Autodesk Inventor part; units mm, degrees
ref_plane "to_base_XY" through (0, -0.0254, 0) normal (0, 1, 0) x (1, 0, 0)
ref_plane "to_base_YZ" through (0, -0.0254, 0) normal (1, 0, 0) x (0, 0, -1)
ref_plane "to_base_ZX" through (0, -0.0254, 0) normal (0, 0, -1) x (0, 1, 0)
sketch "Sketch_2" plane through (0, 0, 0) normal (0, 1, 0) x (-1, 0, 0)
  line L0 (4.7037, -5.0719) -> (4.7037, 5.0719)
  arc A0 (4.7037, 5.0719) -> (4.5737, 5.2019) centre (4.5737, 5.0719) ccw
  line L1 (4.5737, 5.2019) -> (-4.5737, 5.2019)
  arc A1 (-4.5737, 5.2019) -> (-4.7037, 5.0719) centre (-4.5737, 5.0719) ccw
  line L2 (-4.7037, 5.0719) -> (-4.7037, -5.0719)
  arc A2 (-4.7037, -5.0719) -> (-4.5737, -5.2019) centre (-4.5737, -5.0719) ccw
  line L3 (-4.5737, -5.2019) -> (4.5737, -5.2019)
  arc A3 (4.5737, -5.2019) -> (4.7037, -5.0719) centre (4.5737, -5.0719) ccw
extrude "Extrusion1" add sketch "Sketch_2" along normal blind 0.254
sketch "Sketch_1" plane through (0, 0, -4.699) normal (0, 0, 1) x (1, 0, 0)
  line L0 (1.016, 0) -> (1.016, -1.016)
  line L1 (1.016, -1.016) -> (1.27, -1.016)
  line L2 (1.27, -1.016) -> (1.27, -2.4384)
  arc A0 (1.27, -2.4384) -> (2.413, -3.5814) centre (2.413, -2.4384) ccw
  line L3 (2.413, -3.5814) -> (10.0076, -3.5814)
  arc A1 (10.0076, -3.5814) -> (10.0076, -2.3114) centre (10.0076, -2.9464) ccw
  line L4 (10.0076, -2.3114) -> (3.048, -2.3114)
  arc A2 (2.54, -1.8034) -> (3.048, -2.3114) centre (3.048, -1.8034) ccw
  line L5 (2.54, -1.8034) -> (2.54, -1.016)
  line L6 (2.54, -1.016) -> (2.794, -1.016)
  line L7 (2.794, -1.016) -> (2.794, 0)
  line L8 (2.794, 0) -> (1.016, 0)
extrude "Extrusion2" add sketch "Sketch_1" along normal mid plane 0.762
pattern_linear "Rectangular Pattern1" count 3 spacing 4.699 along (0, 0, 1) of "Extrusion2"
sketch "Sketch_18" plane through (0, 0, -4.699) normal (0, 0, 1) x (1, 0, 0)
  line L0 (-2.794, 0) -> (-2.794, -1.016)
  line L1 (-2.794, -1.016) -> (-2.54, -1.016)
  line L2 (-2.54, -1.016) -> (-2.54, -6.3754)
  arc A0 (-2.54, -6.3754) -> (-1.524, -7.3914) centre (-1.524, -6.3754) ccw
  line L3 (-1.524, -7.3914) -> (10.0076, -7.3914)
  arc A1 (10.0076, -7.3914) -> (10.0076, -6.1214) centre (10.0076, -6.7564) ccw
  line L4 (10.0076, -6.1214) -> (-0.762, -6.1214)
  arc A2 (-1.27, -5.6134) -> (-0.762, -6.1214) centre (-0.762, -5.6134) ccw
  line L5 (-1.27, -5.6134) -> (-1.27, -1.016)
  line L6 (-1.27, -1.016) -> (-1.016, -1.016)
  line L7 (-1.016, -1.016) -> (-1.016, 0)
  line L8 (-1.016, 0) -> (-2.794, 0)
extrude "Extrusion3" add sketch "Sketch_18" along normal mid plane 0.762
pattern_linear "Rectangular Pattern2" count 3 spacing 4.699 along (0, 0, 1) of "Extrusion3"
ref_plane "to_base_XY" through (0, -0.0254, 0) normal (0, 1, 0) x (1, 0, 0)
ref_plane "to_base_YZ" through (0, -0.0254, 0) normal (1, 0, 0) x (0, 0, -1)
ref_plane "to_base_ZX" through (0, -0.0254, 0) normal (0, 0, -1) x (0, 1, 0)
properties part number "M202830_terminal_angW"
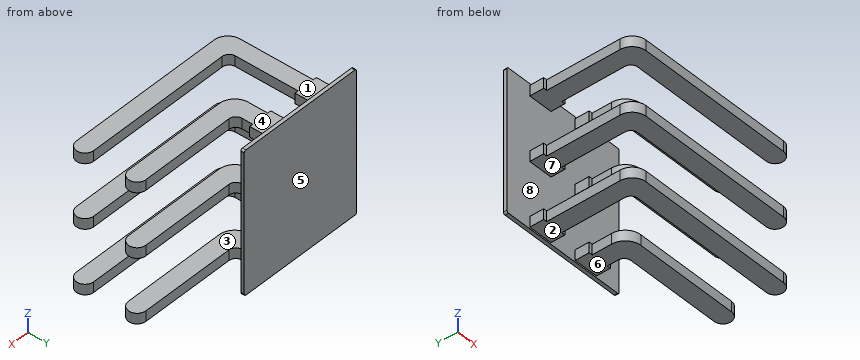
Build history of the part. All positions in model axes, mm. Face numbers are marked on the shaded views. A direction names the side the tool comes from. Coordinates: 2 decimals unless noted, no trailing zeros. Write each loop counter-clockwise with the first axis right and the second up, starting at its lowest first coordinate (ties: lowest second). Pieces come first, ordered by that corner, then holes. Notation, with made-up numbers: (-33.75, -1.75) -> (-20.75, -1.75) arc R18 ccw to (-20.75, 9.25) -> close; hole circle Ø7 at (-20.5, -4). An arc over 180 degrees is marked (long way). Use CSV: the item, a comma, the result in double quotes. Start each with the question number.
Q1. 3-axis set-ups, long thin cutter, end or side, ignore diameter. For the marked faces 4, 5, 6, 7 and 8: which of +Z, -Z, +X, -X, +Y, -Y reach the whole face in a straight line?
Q2. Cut at D-D, the plane z = 4.5. List the corners of the cut face in (x, y) (3 decimals).
Q3. Cut at A-A, the plane y = -5. List the corners of the cut face in (x, z).
Q4. Flat gauge pins, fed straight in: pin 1 Ø0.8 at (y, z) = (-3.5, 4.5) entering from +X; pin 2 Ø4 at (x, y) = (4, -2.5) entering from -Z; pin 3 Ø1 at (y, z) = (-1, -0.5) entering from -X. Where does each tip first touch, or does it go through?
Q5. Cut at C-C, the plane y = -1.5. List the corners of the cut face in (x, z).
Q6. Cut at B-B, the plane x = 9.5. List the corners of the cut face in (y, z), then the cut area to 3 significant figures.
Q7. Pull direction Z, two halves, no side cores. Call the marked faces 1, 2 and 3: released by +Z, released by -Z, zero draft, split by the parting line, or undercut.
Q8. Drill centre lines: probe 1 along Z at (x, y) = (9, -2.5); probe 2 along Y at (x, z) = (6.5, -0.25); probe 3 along Y at (x, z) = (-0.75, 4.5). Where is each one in solid material? Low to high.
Checked values:
1,face 4,"+Z, +X, -X, -Y"
1,face 5,"+Z, -Z, +X, -X, +Y"
1,face 6,"-Z, +X, -X, -Y"
1,face 7,"+X, -X, -Y"
1,face 8,"none"
2,outline,"(-4.704, 0) -> (-2.794, 0) -> (-2.794, -1.016) -> (-2.54, -1.016) -> (-2.54, -6.375) arc R1.016 ccw to (-1.524, -7.391) -> (10.008, -7.391) arc R0.635 ccw to (10.008, -6.121) -> (-0.762, -6.121) arc R0.508 cw to (-1.27, -5.613) -> (-1.27, -1.016) -> (-1.016, -1.016) -> (-1.016, 0) -> (1.016, 0) -> (1.016, -1.016) -> (1.27, -1.016) -> (1.27, -2.438) arc R1.143 ccw to (2.413, -3.581) -> (10.008, -3.581) arc R0.635 ccw to (10.008, -2.311) -> (3.048, -2.311) arc R0.508 cw to (2.54, -1.803) -> (2.54, -1.016) -> (2.794, -1.016) -> (2.794, 0) -> (4.704, 0) -> (4.704, 0.254) -> (-4.704, 0.254) -> close"
3,outline,"(-2.54, -5.08) -> (-1.27, -5.08) -> (-1.27, -4.32) -> (-2.54, -4.32) -> close; (-2.54, -0.38) -> (-1.27, -0.38) -> (-1.27, 0.38) -> (-2.54, 0.38) -> close; (-2.54, 4.32) -> (-1.27, 4.32) -> (-1.27, 5.08) -> (-2.54, 5.08) -> close"
4,pin 1,"stops at x = 10.62"
4,pin 2,"stops at z = -5.08"
4,pin 3,"stops at x = -2.79"
5,outline,"(-2.54, -5.08) -> (-1.27, -5.08) -> (-1.27, -4.32) -> (-2.54, -4.32) -> close; (-2.54, -0.38) -> (-1.27, -0.38) -> (-1.27, 0.38) -> (-2.54, 0.38) -> close; (-2.54, 4.32) -> (-1.27, 4.32) -> (-1.27, 5.08) -> (-2.54, 5.08) -> close; (1.27, -5.08) -> (2.54, -5.08) -> (2.54, -4.32) -> (1.27, -4.32) -> close; (1.27, -0.38) -> (2.54, -0.38) -> (2.54, 0.38) -> (1.27, 0.38) -> close; (1.27, 4.32) -> (2.54, 4.32) -> (2.54, 5.08) -> (1.27, 5.08) -> close"
6,outline,"(-7.39, -5.08) -> (-6.12, -5.08) -> (-6.12, -4.32) -> (-7.39, -4.32) -> close; (-7.39, -0.38) -> (-6.12, -0.38) -> (-6.12, 0.38) -> (-7.39, 0.38) -> close; (-7.39, 4.32) -> (-6.12, 4.32) -> (-6.12, 5.08) -> (-7.39, 5.08) -> close; (-3.58, -5.08) -> (-2.31, -5.08) -> (-2.31, -4.32) -> (-3.58, -4.32) -> close; (-3.58, -0.38) -> (-2.31, -0.38) -> (-2.31, 0.38) -> (-3.58, 0.38) -> close; (-3.58, 4.32) -> (-2.31, 4.32) -> (-2.31, 5.08) -> (-3.58, 5.08) -> close"
6,area,"5.81 mm²"
7,face 1,"released by +Z"
7,face 2,"released by -Z"
7,face 3,"undercut"
8,probe 1,"z = -5.08 to -4.32, -0.38 to 0.38, 4.32 to 5.08"
8,probe 2,"y = -7.39 to -6.12, -3.58 to -2.31"
8,probe 3,"y = -7.39 to -6.12, 0 to 0.25"
